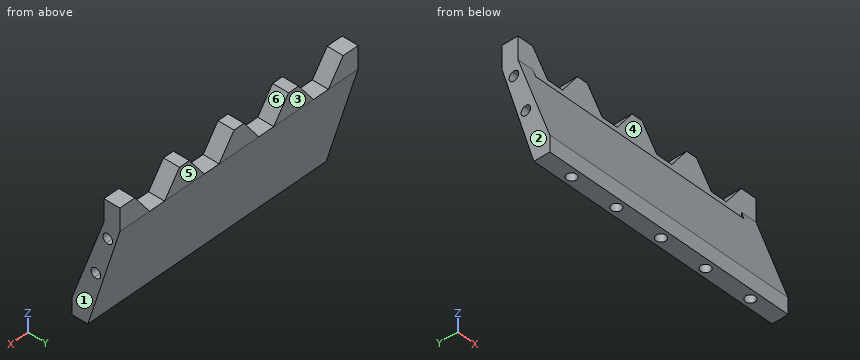
from build123d import *

# Parameters (mm, degrees)
F1_DEPTH  = 6.35
F0_W      = 88.9
F0_H      = 32.385
F2_DEPTH  = 19.05
F5_DEPTH  = 101.6
F6_DEPTH  = 12.7
F9_DEPTH  = 12.7
F11_R     = 1.905
F12_DEPTH = 5.08


# Not quite as in the source:
# - a feature names something its author has since deleted; it is built from what else it names


with BuildPart() as f1:
    # F0 (on Front) → F1 (new body)
    with BuildSketch(Plane.XZ):
        Polygon((50.8, 16.51), (50.8, 25.4), (44.4373, 25.4), (38.0873, 16.51), (31.7373, 16.51), (25.3873, 25.4), (21.1582, 25.4), (14.8082, 16.51), (8.4582, 16.51), (2.1082, 25.4), (-2.1209, 25.4), (-8.4709, 16.51), (-14.8209, 16.51), (-21.1709, 25.4), (-25.4, 25.4), (-31.75, 16.51), (-38.1, 16.51), (-44.45, 25.4), (-50.8, 25.4), (-50.8, 16.51), (-44.45, 16.51), (-44.45, 13.335), (44.45, 13.335), (44.45, 16.51), align=None)
    extrude(amount=F1_DEPTH)

    # F0 (on Front) → F2 (join)
    with BuildSketch(Plane.XZ):
        Polygon((50.8, -25.4), (50.8, 16.51), (44.45, 16.51), (44.45, 13.335), (44.45, -19.05), (-44.45, -19.05), (-44.45, 13.335), (-44.45, 16.51), (-50.8, 16.51), (-50.8, -25.4), (-44.45, -25.4), (44.45, -25.4), align=None)
        with Locations((0, -2.8575)):
            Rectangle(F0_W, F0_H)
    extrude(amount=F2_DEPTH)

    # F4 (on offset) → F5 (cut)
    with BuildSketch(Plane.YZ.offset(50.8)):
        Polygon((-12.7, -25.4), (0, -25.4), (0, 16.51), align=None)
        Polygon((-6.35, 16.51), (-6.35, 25.4), (-19.05, 25.4), (-19.05, -19.05), align=None)
    extrude(amount=-F5_DEPTH, mode=Mode.SUBTRACT)

    # F4 (on offset) → F6 (cut)
    with BuildSketch(Plane.YZ.offset(50.8)):
        with BuildLine():
            ThreePointArc((-8.972535912, -2.6218685096), (-11.3481314904, -3.892535912), (-10.077464088, -6.2681314904))
            ThreePointArc((-10.077464088, -6.2681314904), (-8.3899711651, -5.9749459284), (-7.62, -4.445))
            ThreePointArc((-7.62, -4.445), (-7.9950540716, -3.3099711651), (-8.972535912, -2.6218685096))
        make_face()
        with BuildLine():
            ThreePointArc((-2.897765424, 11.1383741007), (-3.2728194956, 12.2734029356), (-4.250301336, 12.9615055911))
            ThreePointArc((-4.250301336, 12.9615055911), (-6.6258969145, 11.6908381887), (-5.3552295121, 9.3152426102))
            ThreePointArc((-5.3552295121, 9.3152426102), (-3.6677365891, 9.6084281723), (-2.897765424, 11.1383741007))
        make_face()
    extrude(amount=-F6_DEPTH, mode=Mode.SUBTRACT)

    # F8 (on offset) → F9 (cut)
    with BuildSketch(Plane(origin=(-50.8, 0, 0), x_dir=(0, -1, 0), z_dir=(-1, 0, 0))):
        with BuildLine():
            ThreePointArc((4.2333912752, 13.0173087917), (2.9627238728, 10.6417132133), (5.3383194513, 9.3710458109))
            ThreePointArc((5.3383194513, 9.3710458109), (6.3158012916, 10.0591484663), (6.6908553632, 11.1941773013))
            ThreePointArc((6.6908553632, 11.1941773013), (5.9208841982, 12.7241232297), (4.2333912752, 13.0173087917))
        make_face()
        with BuildLine():
            ThreePointArc((8.972535912, -2.6218685096), (7.7018685096, -4.997464088), (10.077464088, -6.2681314904))
            ThreePointArc((10.077464088, -6.2681314904), (11.0549459284, -5.5800288349), (11.43, -4.445))
            ThreePointArc((11.43, -4.445), (10.6600288349, -2.9150540716), (8.972535912, -2.6218685096))
        make_face()
    extrude(amount=-F9_DEPTH, mode=Mode.SUBTRACT)

    # F11 (on offset) → F12 (cut)
    with BuildSketch(Plane(origin=(0, 0, -25.4), x_dir=(1, 0, 0), z_dir=(0, 0, -1))):
        with Locations((-38.1, 15.875)):
            Circle(F11_R)
        with Locations((-19.05, 15.875)):
            Circle(F11_R)
        with Locations((0, 15.875)):
            Circle(F11_R)
        with Locations((19.05, 15.875)):
            Circle(F11_R)
        with Locations((38.1, 15.875)):
            Circle(F11_R)
    extrude(amount=-F12_DEPTH, mode=Mode.SUBTRACT)


solid = f1.part
Source: CAD feature listing. Evaluate the final solid. Frame: model axes, mm. Face numbers are marked on the shaded views. A direction names the side the tool comes from. Give positions to 0.01 mm unless a question says otherwise; leave off trailing zeros. Loops run counter-clockwise (first coordinate to the right, second up) from the corner with the lowest first, then second, coordinate; pieces in that order, holes last. Notation, with made-up numbers: (28.5, 7.25) -> (68.5, 7.25) arc R18 ccw to (68.5, 14.25) -> close; hole circle Ø8 at (-39, 55.25). An arc over 180 degrees is marked (long way). Use a Markdown table: item, result. Add a question column.
1) Section query C-C, the plane x = -33. Return the cut outline in (y, z) (3 decimals), then the cut area to 3 significant figures.
2) Pull-direction query (X, two-part tool) for the marked faces 1, 2, 3 and 4; classes: +X half, -X half, draft (parallel to the pull), parting line (faces both ways), or undercut.
3) Section query D-D, the plane x = 19.05. Return the cut outline in (y, z) (3 decimals).
4) Reachability of the marked faces 5 and 6 from +Z, -Z, +X, -X, +Y, -Y: full face, straight path, thin tool, end or side. Return the list, or none.
5) Section query B-B, the plane x = 0. Return the cut outline in (y, z) (3 decimals), then the cut area to 3 significant figures.
6) First-contact query: pin 1 (3.5 mm diameter, centred on x = 6.5, z = 20.5, fed in from -Y); pin 2 (1.9 mm diameter, centred on x = 10.5, y = -4.5, fed in from +Z); pin 3 (7 mm diameter, centred on x = -11.5, y = -2, fed in from +Z). Flat tips, straight axial feed; report the tip coordinate or a pass-through.
7) Line query: line 1 along Y through (x, z) = (-38.1, -21.65); line 2 along X through (y, z) = (-8.25, -4); line 3 along Y through (x, z) = (0, -22.4). Output: solid intervals per line, ascending. Write a range as [from, to].
8) Section query A-A, the plane z = 21. Return the cut outline in (x, y).
Numbers:
| question | item | result |
|---|---|---|
| 1 | outline | (-19.05, -25.4) -> (-12.7, -25.4) -> (0, 16.51) -> (-6.35, 16.51) -> (-6.35, 13.335) -> (-7.484, 13.335) -> (-19.05, -19.05) -> close |
| 1 | area | 305 mm2 |
| 2 | face 1 | +X half |
| 2 | face 2 | -X half |
| 2 | face 3 | draft |
| 2 | face 4 | undercut |
| 3 | outline | (-19.05, -25.4) -> (-17.78, -25.4) -> (-17.78, -20.32) -> (-13.97, -20.32) -> (-13.97, -25.4) -> (-12.7, -25.4) -> (0, 16.51) -> (0, 22.449) -> (-6.35, 22.449) -> (-6.35, 13.335) -> (-7.484, 13.335) -> (-19.05, -19.05) -> close |
| 4 | face 5 | +Z, -Z, +X, -X, +Y |
| 4 | face 6 | +Z, +Y, -Y |
| 5 | outline | (-19.05, -25.4) -> (-17.78, -25.4) -> (-17.78, -20.32) -> (-13.97, -20.32) -> (-13.97, -25.4) -> (-12.7, -25.4) -> (0, 16.51) -> (0, 25.4) -> (-6.35, 25.4) -> (-6.35, 13.335) -> (-7.484, 13.335) -> (-19.05, -19.05) -> close |
| 5 | area | 342 mm2 |
| 6 | pin 1 | stops at y = -6.35 |
| 6 | pin 2 | stops at z = 16.51 |
| 6 | pin 3 | stops at z = 17.17 |
| 7 | line 1 | y = [-19.05, -17.78], [-13.97, -11.56] |
| 7 | line 2 | x = [-38.1, 38.1] |
| 7 | line 3 | y = [-19.05, -17.78], [-13.97, -11.79] |
| 8 | outline | (-50.8, -6.35) -> (-41.31, -6.35) -> (-41.31, 0) -> (-50.8, 0) -> close; (-28.54, -6.35) -> (-18.03, -6.35) -> (-18.03, 0) -> (-28.54, 0) -> close; (-5.26, -6.35) -> (5.25, -6.35) -> (5.25, 0) -> (-5.26, 0) -> close; (18.02, -6.35) -> (28.53, -6.35) -> (28.53, 0) -> (18.02, 0) -> close; (41.29, -6.35) -> (50.8, -6.35) -> (50.8, 0) -> (41.29, 0) -> close |
